from build123d import *

# Parameters (mm, degrees)
F0_R        = 13.25
F0_R_2      = 11.1
F1_DEPTH    = 3
F2_START    = 1.9
F2_DEPTH    = 1.6
F3_START    = -1.9
F3_DEPTH    = 1.6
F5_D        = 22.2
F6_C1_SIZE  = 0.5
F6_C2_SIZE  = 0.5
F6_C3_SIZE  = 0.4999
F6_C4_SIZE  = 0.4999
F6_C5_SIZE  = 0.4999
F6_C6_SIZE  = 0.4999
F6_C7_SIZE  = 0.4996
F6_C8_SIZE  = 0.5
F6_C9_SIZE  = 0.4999
F6_C10_SIZE = 0.5
F6_C11_SIZE = 0.5
F6_C12_SIZE = 0.4999
F6_C13_SIZE = 0.4996
F6_C14_SIZE = 0.5


# Not quite as in the source:
# - a fillet or chamfer is up to 0.001 mm smaller than in the source, because OpenCascade refuses the exact size


with BuildPart() as f1:
    # F0 (on Front) → F1 (new body, symmetric)
    with BuildSketch(Plane.XZ):
        with BuildLine():
            ThreePointArc((20.4544666255, 0.9003555386), (12.301399045, 7.10221605), (11.0069640816, 17.2639099492))
            ThreePointArc((11.0069640816, 17.2639099492), (0, 42.4544321001), (-11.0069640816, 17.2639099492))
            ThreePointArc((-11.0069640816, 17.2639099492), (-12.301399045, 7.10221605), (-20.4544666255, 0.9003555386))
            ThreePointArc((-20.4544666255, 0.9003555386), (-36.7666167019, -21.22721605), (-9.4475025439, -18.1642654878))
            ThreePointArc((-9.4475025439, -18.1642654878), (0, -14.2044321001), (9.4475025439, -18.1642654878))
            ThreePointArc((9.4475025439, -18.1642654878), (36.7666167019, -21.22721605), (20.4544666255, 0.9003555386))
        make_face()
        with Locations((-23.7762356451, -13.72721605)):
            Circle(F0_R, mode=Mode.SUBTRACT)
        with Locations((23.7762356451, -13.72721605)):
            Circle(F0_R, mode=Mode.SUBTRACT)
        Circle(F0_R_2, mode=Mode.SUBTRACT)
        with Locations((0, 27.4544321001)):
            Circle(F0_R, mode=Mode.SUBTRACT)
    extrude(amount=F1_DEPTH, both=True)

    # F0 (on Front) → F2 (join)
    with BuildSketch(Plane.XZ.offset(F2_START)):
        with BuildLine():
            ThreePointArc((20.4544666255, 0.9003555386), (12.301399045, 7.10221605), (11.0069640816, 17.2639099492))
            ThreePointArc((11.0069640816, 17.2639099492), (0, 42.4544321001), (-11.0069640816, 17.2639099492))
            ThreePointArc((-11.0069640816, 17.2639099492), (-12.301399045, 7.10221605), (-20.4544666255, 0.9003555386))
            ThreePointArc((-20.4544666255, 0.9003555386), (-36.7666167019, -21.22721605), (-9.4475025439, -18.1642654878))
            ThreePointArc((-9.4475025439, -18.1642654878), (0, -14.2044321001), (9.4475025439, -18.1642654878))
            ThreePointArc((9.4475025439, -18.1642654878), (36.7666167019, -21.22721605), (20.4544666255, 0.9003555386))
        make_face()
        with Locations((-23.7762356451, -13.72721605)):
            Circle(F0_R, mode=Mode.SUBTRACT)
        with Locations((23.7762356451, -13.72721605)):
            Circle(F0_R, mode=Mode.SUBTRACT)
        Circle(F0_R_2, mode=Mode.SUBTRACT)
        with Locations((0, 27.4544321001)):
            Circle(F0_R, mode=Mode.SUBTRACT)
        with Locations((-23.7762356451, -13.72721605)):
            Circle(F0_R)
        with Locations((0, 27.4544321001)):
            Circle(F0_R)
        with Locations((23.7762356451, -13.72721605)):
            Circle(F0_R)
        Circle(F0_R_2)
    extrude(amount=F2_DEPTH)

    # F0 (on Front) → F3 (join)
    with BuildSketch(Plane.XZ.offset(F3_START)):
        with BuildLine():
            ThreePointArc((20.4544666255, 0.9003555386), (12.301399045, 7.10221605), (11.0069640816, 17.2639099492))
            ThreePointArc((11.0069640816, 17.2639099492), (0, 42.4544321001), (-11.0069640816, 17.2639099492))
            ThreePointArc((-11.0069640816, 17.2639099492), (-12.301399045, 7.10221605), (-20.4544666255, 0.9003555386))
            ThreePointArc((-20.4544666255, 0.9003555386), (-36.7666167019, -21.22721605), (-9.4475025439, -18.1642654878))
            ThreePointArc((-9.4475025439, -18.1642654878), (0, -14.2044321001), (9.4475025439, -18.1642654878))
            ThreePointArc((9.4475025439, -18.1642654878), (36.7666167019, -21.22721605), (20.4544666255, 0.9003555386))
        make_face()
        with Locations((-23.7762356451, -13.72721605)):
            Circle(F0_R, mode=Mode.SUBTRACT)
        with Locations((23.7762356451, -13.72721605)):
            Circle(F0_R, mode=Mode.SUBTRACT)
        Circle(F0_R_2, mode=Mode.SUBTRACT)
        with Locations((0, 27.4544321001)):
            Circle(F0_R, mode=Mode.SUBTRACT)
        with Locations((0, 27.4544321001)):
            Circle(F0_R)
        with Locations((-23.7762356451, -13.72721605)):
            Circle(F0_R)
        with Locations((23.7762356451, -13.72721605)):
            Circle(F0_R)
        Circle(F0_R_2)
    extrude(amount=-F3_DEPTH)

    # F5 (through all)
    with Locations(Plane.XZ.offset(3.5)):
        with Locations((0, 0)):
            Hole(F5_D / 2)

    # F6: chamfer of 0.5 on 14 edges, made by hand

    # F6_c1
    f6_c1_edges = [f1.edges().sort_by_distance(p)[0] for p in [
        (12.301399045, 3.5, 7.10221605),
    ]]
    chamfer(f6_c1_edges, length=F6_C1_SIZE)

    # F6_c2
    f6_c2_edges = [f1.edges().sort_by_distance(p)[0] for p in [
        (12.301399045, -3.5, 7.10221605),
    ]]
    chamfer(f6_c2_edges, length=F6_C2_SIZE)

    # F6_c3 (size 0.5 in the source; OpenCascade refuses exactly that, so slightly less here)
    f6_c3_edges = [f1.edges().sort_by_distance(p)[0] for p in [
        (36.7666167019, 3.5, -21.22721605),
    ]]
    chamfer(f6_c3_edges, length=F6_C3_SIZE)

    # F6_c4 (size 0.5 in the source; OpenCascade refuses exactly that, so slightly less here)
    f6_c4_edges = [f1.edges().sort_by_distance(p)[0] for p in [
        (0, 3.5, 42.4544321001),
    ]]
    chamfer(f6_c4_edges, length=F6_C4_SIZE)

    # F6_c5 (size 0.5 in the source; OpenCascade refuses exactly that, so slightly less here)
    f6_c5_edges = [f1.edges().sort_by_distance(p)[0] for p in [
        (0, 3.5, -14.2044321001),
    ]]
    chamfer(f6_c5_edges, length=F6_C5_SIZE)

    # F6_c6 (size 0.5 in the source; OpenCascade refuses exactly that, so slightly less here)
    f6_c6_edges = [f1.edges().sort_by_distance(p)[0] for p in [
        (-12.301399045, 3.5, 7.10221605),
    ]]
    chamfer(f6_c6_edges, length=F6_C6_SIZE)

    # F6_c7 (size 0.5 in the source; OpenCascade refuses exactly that, so slightly less here)
    f6_c7_edges = [f1.edges().sort_by_distance(p)[0] for p in [
        (-36.7666167019, 3.5, -21.22721605),
    ]]
    chamfer(f6_c7_edges, length=F6_C7_SIZE)

    # F6_c8
    f6_c8_edges = [f1.edges().sort_by_distance(p)[0] for p in [
        (-11.1, 3.5, 0),
    ]]
    chamfer(f6_c8_edges, length=F6_C8_SIZE)

    # F6_c9 (size 0.5 in the source; OpenCascade refuses exactly that, so slightly less here)
    f6_c9_edges = [f1.edges().sort_by_distance(p)[0] for p in [
        (0, -3.5, 42.4544321001),
    ]]
    chamfer(f6_c9_edges, length=F6_C9_SIZE)

    # F6_c10
    f6_c10_edges = [f1.edges().sort_by_distance(p)[0] for p in [
        (36.7666167019, -3.5, -21.22721605),
    ]]
    chamfer(f6_c10_edges, length=F6_C10_SIZE)

    # F6_c11
    f6_c11_edges = [f1.edges().sort_by_distance(p)[0] for p in [
        (0, -3.5, -14.2044321001),
    ]]
    chamfer(f6_c11_edges, length=F6_C11_SIZE)

    # F6_c12 (size 0.5 in the source; OpenCascade refuses exactly that, so slightly less here)
    f6_c12_edges = [f1.edges().sort_by_distance(p)[0] for p in [
        (-12.301399045, -3.5, 7.10221605),
    ]]
    chamfer(f6_c12_edges, length=F6_C12_SIZE)

    # F6_c13 (size 0.5 in the source; OpenCascade refuses exactly that, so slightly less here)
    f6_c13_edges = [f1.edges().sort_by_distance(p)[0] for p in [
        (-36.7666167019, -3.5, -21.22721605),
    ]]
    chamfer(f6_c13_edges, length=F6_C13_SIZE)

    # F6_c14
    f6_c14_edges = [f1.edges().sort_by_distance(p)[0] for p in [
        (-11.1, -3.5, 0),
    ]]
    chamfer(f6_c14_edges, length=F6_C14_SIZE)


solid = f1.part
Can you work these out from the model? Positions are in its coordinate system, mm. A direction names the side the tool comes from. Coordinates: 2 decimals unless noted, no trailing zeros. Loops run counter-clockwise (first coordinate to the right, second up) from the corner with the lowest first, then second, coordinate; pieces in that order, holes last. Notation, with made-up numbers: (70, 83) - (86, 83) arc R11 cw to (86, 104) - close; hole circle Ø10 at (8, 59). An arc over 180 degrees is marked (long way). Put each result on its own line as item: value. Start each with the question number.
Item 1: If I drill on line 1 along X through (y, z) = (0.5, -12.5); line 2 along Z through (x, y) = (0, 2.8); line 3 along Z through (x, y) = (-23.5, 0.5), over which ranges is the centre line in solid material (lowest first)?
Item 2: If we mould it in two halves opening along Z, with no side actions, what happens to faces 3 (the face through (-0.15, 3.135, -14.07)), 4 (the face through (-36.21, 3.36, -21.46)), 5 (the face through (24, -1.9, -14))? For each: +Z half, -Z half, draft (parallel to the pull), parting line (faces both ways), or undercut.
Item 3: Suppose I cut it at B-B (z = -20.5). State how many separate pieces and enclosed holes the cut face has, and give its area (3 significant figures).
Item 4: For pin 1 (4 mm diameter, centred on y = 1, z = -2.5, fed in from +X); pin 2 (4 mm diameter, centred on x = -3.5, y = -2.5, fed in from +Z); pin 3 (18 mm diameter, centred on x = 0, z = 0, fed in from -Y); pin 4 (3 mm diameter, centred on x = 20, y = 1, fed in from +Z), each with a flat end and sliding along its axis, tell me the tip position at first contact or that it passes through.
Item 5: Which directions (+Z, -Z, +X, -X, +Y, -Y) give clear straight access to the entire face, cutting with the end or side of a thin tool? Please do faces 1 (the face through (0.477, 3.358, 42.089)), 2 (the face through (24, 1.9, -14)).
Item 6: Suppose I cut it at A-A (x = 0). Please give me the cut outline in (y, z), and give its area (3 significant figures).
Here are the results:
1. line 1: -38.73 to -36.97, -10.58 to 10.58, 36.97 to 38.73
1. line 2: -14.2 to -11.1, 11.1 to 42.45
1. line 3: -28.72 to -26.97, -0.48 to 1.27
2. face 3: -Z half
2. face 4: parting line
2. face 5: undercut
3. separate pieces: 2
3. enclosed holes: 2
3. area: 201 mm²
4. pin 1: x = 35.6
4. pin 2: z = 42.38
4. pin 3: through
4. pin 4: z = 1.57
5. face 1: +Y
5. face 2: none
6. outline: (-3.5, -13.7) - (-3, -14.2) - (3, -14.2) - (3.5, -13.7) - (3.5, -11.6) - (3, -11.1) - (-3, -11.1) - (-3.5, -11.6) - close; (-3.5, 11.6) - (-3, 11.1) - (3, 11.1) - (3.5, 11.6) - (3.5, 41.95) - (3, 42.45) - (-3, 42.45) - (-3.5, 41.95) - close; hole (-1.9, 14.2) - (1.9, 14.2) - (1.9, 40.7) - (-1.9, 40.7) - close
6. area: 140 mm²
